from build123d import *

# Parameters (mm, degrees)
SKETCH1_W           = 89.98
SKETCH1_H           = 32
SKETCH1_R           = 4
SKETCH1_R_2         = 1.25
BOSS_EXTRUDE1_DEPTH = 3
BOSS_EXTRUDE2_START = 3
SKETCH1_5_R         = 4
SKETCH1_5_R_2       = 1.25
BOSS_EXTRUDE2_DEPTH = 1
BOSS_EXTRUDE3_START = 4
BOSS_EXTRUDE3_DEPTH = 1.6
SKETCH2_W           = 90.38
SKETCH2_H           = 1.5
BOSS_EXTRUDE4_DEPTH = 1


with BuildPart() as part:
    # Sketch1 → Boss-Extrude1 (new body)
    # profile 1 of 5: a face of its own
    with BuildSketch(Plane(origin=(0, 0, 0), x_dir=(1, 0, 0), z_dir=(0, 1, 0))):
        with Locations((44.99, -16)):
            Rectangle(SKETCH1_W, SKETCH1_H)
        with Locations((78.98, -9.5)):
            Circle(SKETCH1_R, mode=Mode.SUBTRACT)
        with Locations((11, -9.5)):
            Circle(SKETCH1_R, mode=Mode.SUBTRACT)
    # profile 2 of 5: a face of its own
    with BuildSketch(Plane(origin=(0, 0, 0), x_dir=(1, 0, 0), z_dir=(0, 1, 0))):
        with Locations((11, -9.5)):
            Circle(SKETCH1_R)
        with Locations(Location((11, -9.5, 0), (0, 0, 270))):
            Circle(SKETCH1_R_2, mode=Mode.SUBTRACT)
    # profile 3 of 5: a face of its own
    with BuildSketch(Plane(origin=(0, 0, 0), x_dir=(1, 0, 0), z_dir=(0, 1, 0))):
        Polygon((90.18, -32), (89.98, -32), (89.98, 0), (0, 0), (0, -32), (-0.2, -32), (-0.2, 0.2), (90.18, 0.2), align=None)
    # profile 4 of 5: a face of its own
    with BuildSketch(Plane(origin=(0, 0, 0), x_dir=(1, 0, 0), z_dir=(0, 1, 0))):
        with BuildLine():
            ThreePointArc((-2.2, -32), (-3.614213562, -31.414213562), (-4.2, -30))
            Line((-4.2, -30), (-4.2, 1))
            ThreePointArc((-4.2, 1), (-3.321320344, 3.121320344), (-1.2, 4))
            Line((-1.2, 4), (91.18, 4))
            ThreePointArc((91.18, 4), (93.301320344, 3.121320344), (94.18, 1))
            Line((94.18, 1), (94.18, -30))
            ThreePointArc((94.18, -30), (93.594213562, -31.414213562), (92.18, -32))
            Line((92.18, -32), (90.18, -32))
            Line((90.18, -32), (90.18, 0.2))
            Line((90.18, 0.2), (-0.2, 0.2))
            Line((-0.2, 0.2), (-0.2, -32))
            Line((-0.2, -32), (-2.2, -32))
        make_face()
    # profile 5 of 5: a face of its own
    with BuildSketch(Plane(origin=(0, 0, 0), x_dir=(1, 0, 0), z_dir=(0, 1, 0))):
        with Locations((78.98, -9.5)):
            Circle(SKETCH1_R)
        with Locations(Location((78.98, -9.5, 0), (0, 0, 270))):
            Circle(SKETCH1_R_2, mode=Mode.SUBTRACT)
    extrude(amount=BOSS_EXTRUDE1_DEPTH)

    # Sketch1<5> → Boss-Extrude2 (add)
    # profile 1 of 3: a face of its own
    with BuildSketch(Plane(origin=(0, 0, 0), x_dir=(1, 0, 0), z_dir=(0, 1, 0)).offset(BOSS_EXTRUDE2_START)):
        with Locations(Location((11, -9.5, 0), (0, 0, 270))):
            Circle(SKETCH1_5_R)
        with Locations(Location((11, -9.5, 0), (0, 0, 270))):
            Circle(SKETCH1_5_R_2, mode=Mode.SUBTRACT)
    # profile 2 of 3: a face of its own
    with BuildSketch(Plane(origin=(0, 0, 0), x_dir=(1, 0, 0), z_dir=(0, 1, 0)).offset(BOSS_EXTRUDE2_START)):
        with BuildLine():
            ThreePointArc((-2.2, -32), (-3.614213562, -31.414213562), (-4.2, -30))
            Line((-4.2, -30), (-4.2, 1))
            ThreePointArc((-4.2, 1), (-3.321320344, 3.121320344), (-1.2, 4))
            Line((-1.2, 4), (91.18, 4))
            ThreePointArc((91.18, 4), (93.301320344, 3.121320344), (94.18, 1))
            Line((94.18, 1), (94.18, -30))
            ThreePointArc((94.18, -30), (93.594213562, -31.414213562), (92.18, -32))
            Line((92.18, -32), (90.18, -32))
            Line((90.18, -32), (90.18, 0.2))
            Line((90.18, 0.2), (-0.2, 0.2))
            Line((-0.2, 0.2), (-0.2, -32))
            Line((-0.2, -32), (-2.2, -32))
        make_face()
    # profile 3 of 3: a face of its own
    with BuildSketch(Plane(origin=(0, 0, 0), x_dir=(1, 0, 0), z_dir=(0, 1, 0)).offset(BOSS_EXTRUDE2_START)):
        with Locations(Location((78.98, -9.5, 0), (0, 0, 270))):
            Circle(SKETCH1_5_R)
        with Locations(Location((78.98, -9.5, 0), (0, 0, 270))):
            Circle(SKETCH1_5_R_2, mode=Mode.SUBTRACT)
    extrude(amount=BOSS_EXTRUDE2_DEPTH)

    # Sketch1<6> → Boss-Extrude3 (add)
    with BuildSketch(Plane(origin=(0, 0, 0), x_dir=(1, 0, 0), z_dir=(0, 1, 0)).offset(BOSS_EXTRUDE3_START)):
        with BuildLine():
            ThreePointArc((-2.2, -32), (-3.614213562, -31.414213562), (-4.2, -30))
            Line((-4.2, -30), (-4.2, 1))
            ThreePointArc((-4.2, 1), (-3.321320344, 3.121320344), (-1.2, 4))
            Line((-1.2, 4), (91.18, 4))
            ThreePointArc((91.18, 4), (93.301320344, 3.121320344), (94.18, 1))
            Line((94.18, 1), (94.18, -30))
            ThreePointArc((94.18, -30), (93.594213562, -31.414213562), (92.18, -32))
            Line((92.18, -32), (90.18, -32))
            Line((90.18, -32), (90.18, 0.2))
            Line((90.18, 0.2), (-0.2, 0.2))
            Line((-0.2, 0.2), (-0.2, -32))
            Line((-0.2, -32), (-2.2, -32))
        make_face()
    extrude(amount=BOSS_EXTRUDE3_DEPTH)

    # Sketch2 → Boss-Extrude4 (add)
    with BuildSketch(Plane(origin=(0, 3, 0), x_dir=(1, 0, 0), z_dir=(0, 1, 0))):
        with Locations((44.99, -31.25)):
            Rectangle(SKETCH2_W, SKETCH2_H)
    extrude(amount=BOSS_EXTRUDE4_DEPTH)


solid = part.part
For this review, take the finished solid that the model builds, in its own axes (mm). A direction names the side the tool comes from. Give positions to 0.01 mm unless a question says otherwise; leave off trailing zeros. Loops run counter-clockwise (first coordinate to the right, second up) from the corner with the lowest first, then second, coordinate; pieces in that order, holes last. Notation, with made-up numbers: (59.25, 26.5) -> (79.25, 26.5) arc R29 ccw to (79.25, 64.5) -> close; hole circle Ø2 at (81, 16). An arc over 180 degrees is marked (long way). One line per question, with ' | ' between items.
1) To check wall thickness, follow probe 1 along X at (y, z) = (2.6, 9.5); probe 2 along X at (y, z) = (4.25, 29); probe 3 along Z at (x, y) = (78.98, 2). State the ranges of each line that lie inside material, in increasing order.
Resolved:
probe 1: x = -4.2 to 9.75, 12.25 to 77.73, 80.23 to 94.18 | probe 2: x = -4.2 to -0.2, 90.18 to 94.18 | probe 3: z = -4 to 8.25, 10.75 to 32
2) We need section A-A (x = 11). Write out the cut boundary in (y, z).
Resolved:
outline: (0, -4) -> (5.6, -4) -> (5.6, -0.2) -> (3, -0.2) -> (3, 5.5) -> (4, 5.5) -> (4, 8.25) -> (0, 8.25) -> close; (0, 10.75) -> (4, 10.75) -> (4, 13.5) -> (3, 13.5) -> (3, 30.5) -> (4, 30.5) -> (4, 32) -> (0, 32) -> close
3) We need section B-B (z = 9.5). Write out the cut boundary in (x, y), plus the area to 3 significant figures.
Resolved:
outline: (-4.2, 0) -> (9.75, 0) -> (9.75, 4) -> (7, 4) -> (7, 3) -> (-0.2, 3) -> (-0.2, 5.6) -> (-4.2, 5.6) -> close; (12.25, 0) -> (77.73, 0) -> (77.73, 4) -> (74.98, 4) -> (74.98, 3) -> (15, 3) -> (15, 4) -> (12.25, 4) -> close; (80.23, 0) -> (94.18, 0) -> (94.18, 5.6) -> (90.18, 5.6) -> (90.18, 3) -> (82.98, 3) -> (82.98, 4) -> (80.23, 4) -> close | area: 312 mm2
4) The part is to be moulded in two halves that separate along Z. For faces 4 (the cylindrical face through (93.61, 2.76, 31.4)), 5 (the flat face through (44, 3, 15)), 6 (the cylindrical face through (-3.34, 2.76, -3.1)), 7 (the flat face through (94.18, 3, 14)), say which applies: +Z half, -Z half, draft (parallel to the pull), parting line (faces both ways), or undercut.
Resolved:
face 4: +Z half | face 5: undercut | face 6: -Z half | face 7: draft
5) We need section C-C (z = 4.5). Write out the cut boundary in (x, y).
Resolved:
outline: (-4.2, 0) -> (94.18, 0) -> (94.18, 5.6) -> (90.18, 5.6) -> (90.18, 3) -> (-0.2, 3) -> (-0.2, 5.6) -> (-4.2, 5.6) -> close
6) We need section D-D (x = 60). Write out the cut boundary in (y, z), plus the area to 3 significant figures.
Resolved:
outline: (0, -4) -> (5.6, -4) -> (5.6, -0.2) -> (3, -0.2) -> (3, 30.5) -> (4, 30.5) -> (4, 32) -> (0, 32) -> close | area: 119 mm2
7) For faces 1 (the flat face through (44, 0, 14)), 2 (the flat face through (79, 4, 11)), 3 (the cylindrical face through (13.7, 3.49, 6.55)), list the 3-axis set-ups (+Z, -Z, +X, -X, +Y, -Y) from which the entire face can be reached by the end or side of a thin tool; tool diameter is ignored.
Resolved:
face 1: +Z, -Z, +X, -X, -Y | face 2: +Z, +Y | face 3: +Y
8) Insertion check: pin 1 Ø9 at (x, z) = (9.5, 9.5) entering from +Y; pin 2 Ø0.8 at (x, y) = (35.5, 5) entering from +Z. Each pin has a flat end and moves straight along its axis. Give the tip position at first contact, or say it passes through.
Resolved:
pin 1: stops at y = 4 | pin 2: stops at z = -0.2
